Could you check a few things on this model? Use its own coordinates, in mm. Give positions to 0.01 mm unless a question says otherwise; leave off trailing zeros. Write each loop counter-clockwise with the first axis right and the second up, starting at its lowest first coordinate (ties: lowest second). Pieces come first, ordered by that corner, then holes. Notation, with made-up numbers: (69.5, 79) -> (114.5, 79) arc R21 ccw to (114.5, 84) -> close; hole circle Ø5 at (71, -15.5). An arc over 180 degrees is marked (long way). One line per question, with ' | ' between items.
from build123d import *

# Parameters (mm, degrees)
SKETCH_1_R      = 46
SKETCH_1_R_2    = 1.5
EXTRUDE_1_DEPTH = 29
FILLET_1_R      = 10
FILLET_2_R      = 10


with BuildPart() as part:
    # 草图1 → 凸台-拉伸1 (new body)
    with BuildSketch(Plane.XY):
        with Locations(Location((0, 0, 0), (0, 0, 180))):
            Circle(SKETCH_1_R)
        with Locations(Location((0, -15.5, 0), (0, 0, 180))):
            Circle(SKETCH_1_R_2, mode=Mode.SUBTRACT)
        with Locations(Location((-15.5, 0, 0), (0, 0, 180))):
            Circle(SKETCH_1_R_2, mode=Mode.SUBTRACT)
        with Locations(Location((0, 15.5, 0), (0, 0, 180))):
            Circle(SKETCH_1_R_2, mode=Mode.SUBTRACT)
        with Locations(Location((15.5, 0, 0), (0, 0, 180))):
            Circle(SKETCH_1_R_2, mode=Mode.SUBTRACT)
    extrude(amount=EXTRUDE_1_DEPTH)

    # 圆角1
    fillet_1_edges = [part.edges().sort_by_distance(p)[0] for p in [
        (46, 0, 29),
    ]]
    fillet(fillet_1_edges, radius=FILLET_1_R)

    # 圆角2
    fillet_2_edges = [part.edges().sort_by_distance(p)[0] for p in [
        (46, 0, 0),
    ]]
    fillet(fillet_2_edges, radius=FILLET_2_R)


solid = part.part
Q1. Will these pins go through, and if not, where does the flat tip stop? pin 1 (4 mm diameter, centred on x = -25.5, z = 7.5, fed in from -Y); pin 2 (12 mm diameter, centred on x = -3, z = 10.5, fed in from +Y); pin 3 (5 mm diameter, centred on y = 22.5, z = 5.5, fed in from -X).
Answer below:
pin 1: stops at y = -39.28 | pin 2: stops at y = 46 | pin 3: stops at x = -40.66
Q2. Imagine slicing it at D-D on z = 25.75. Please give me the cut outline in (x, y), and give its area (3 significant figures).
Answer below:
outline: circle Ø86.76 at (0, 0); hole circle Ø3 at (-15.5, 0); hole circle Ø3 at (0, -15.5); hole circle Ø3 at (0, 15.5); hole circle Ø3 at (15.5, 0) | area: 5,880 mm^2
Q3. If I drill on line 1 along Y through (x, z) = (0, 11.5); line 2 along Y through (x, z) = (0, 21.25); line 3 along X through (y, z) = (-15.5, 15), over which ranges is the centre line in solid material (lowest first)?
Answer below:
line 1: y = -46 to -17, -14 to 14, 17 to 46 | line 2: y = -45.74 to -17, -14 to 14, 17 to 45.74 | line 3: x = -43.31 to -1.5, 1.5 to 43.31
Q4. Imagine slicing it at A-A on y = 0. Please give me the cut outline in (x, z).
Answer below:
outline: (-46, 10) arc R10 ccw to (-36, 0) -> (-17, 0) -> (-17, 29) -> (-36, 29) arc R10 ccw to (-46, 19) -> close; (-14, 0) -> (14, 0) -> (14, 29) -> (-14, 29) -> close; (17, 0) -> (36, 0) arc R10 ccw to (46, 10) -> (46, 19) arc R10 ccw to (36, 29) -> (17, 29) -> close
Q5. If we mould it in two halves opening along Y, with no side actions, what happens to faces 1 (the cylindrical face through (5.99, -45.61, 14.44)), 2 (the cylindrical face through (1.11, -16.51, 14.3)), 3 (the cylindrical face through (17, 0, 14)), 4 (the flat face through (1, -1, 0))? For each: +Y half, -Y half, draft (parallel to the pull), parting line (faces both ways), or undercut.
Answer below:
face 1: parting line | face 2: undercut | face 3: undercut | face 4: draft
Q6. Imagine slicing it at B-B on z = 16.25. Please give me the cut outline in (x, y).
Answer below:
outline: circle Ø92 at (0, 0); hole circle Ø3 at (-15.5, 0); hole circle Ø3 at (0, -15.5); hole circle Ø3 at (0, 15.5); hole circle Ø3 at (15.5, 0)
